Autodesk Fusion 360 part; units mm, degrees
sketch "Esquisse1" plane through (0, 0, 0) normal (0, 0, 1) x (1, 0, 0)
  line L0 (4.3054, 30) -> (67.3054, 30)
  line L1 (67.3054, 30) -> (67.3054, 12.25)
  line L2 (67.3054, 12.25) -> (4.3054, 12.25)
  line L3 (4.3054, 12.25) -> (4.3054, 30)
  dimension "d1" = 63
  dimension "d2" = 17.75
extrude "Extrusion1" add sketch "Esquisse1" along normal blind 1
sketch "Esquisse2" plane through (0, 0, 1) normal (0, 0, 1) x (-1, 0, 0)
  line L0 (-4.3054, -12.25) -> (-67.3054, -12.25)
  line L1 (-67.3054, -12.25) -> (-67.3054, -30)
  line L2 (-67.3054, -30) -> (-4.3054, -30)
  line L3 (-4.3054, -30) -> (-4.3054, -12.25)
  line L4 (-4.3054, -12.95) -> (-6.3054, -12.95)
  line L5 (-6.3054, -12.95) -> (-6.3054, -29.3)
  line L6 (-6.3054, -29.3) -> (-4.3054, -29.3)
  line L7 (-4.3054, -29.3) -> (-4.3054, -12.95)
  line L8 (-67.3054, -21.125) -> (-4.3054, -21.125) construction
  dimension "d5" = 16.35
  dimension "d8" = 2
extrude "Extrusion2" add sketch "Esquisse2" along normal blind 1 contours L3 L4 L5 L6 L7
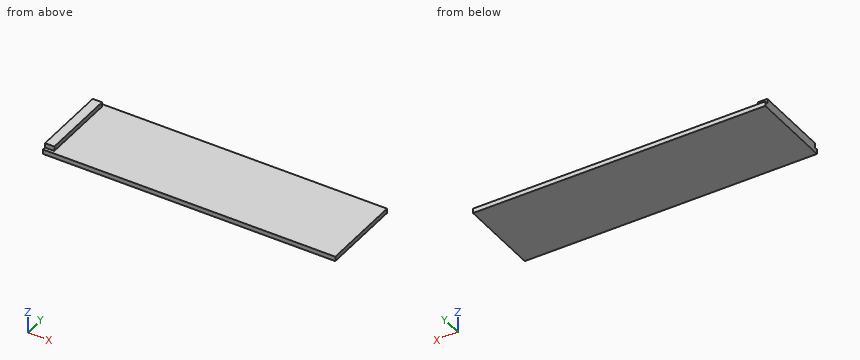
Geometry check sheet. Reference: the model listing, model coordinates, mm. Round coordinates to 2 decimals unless told otherwise and drop trailing zeros. Loops run counter-clockwise (first coordinate to the right, second up) from the corner with the lowest first, then second, coordinate; pieces in that order, holes last. Notation, with made-up numbers: (-14, 62.5) - (-6, 62.5) arc R32 ccw to (-6, 94.5) - close; hole circle Ø5 at (64, 36.25). An arc over 180 degrees is marked (long way). One line per question, with ' | ' between items. Start each with the question number.
1. Cross-section at C-C on x = 29. Record the cut outline in (y, z), then the cut area to 4 significant figures.
2. Depth check by flat-ended pin: pin 1 (0.8 mm diameter, centred on y = 20.5, z = 1.5, fed in from +X); pin 2 (9 mm diameter, centred on x = 44.5, y = 20, fed in from +Z); pin 3 (0.8 mm diameter, centred on x = 5.5, z = 1.5, fed in from +Y). Enter the tip coordinate at first touch or a pass-through.
3. Scan lines: line 1 (Z direction, x = 35, y = 27.75); line 2 (X direction, y = 15.25, z = 1.2). Record each from-to range of solid material in increasing order. Write a range as [from, to].
4. Cross-section at A-A on y = 13.5. Record the cut outline in (x, z).
5. Cross-section at B-B on z = 1.3. Record the cut outline in (x, y).
Taken from the geometry:
1) outline: (12.25, 0) - (30, 0) - (30, 1) - (12.25, 1) - close | area: 17.75 mm²
2) pin 1: x = 6.31 | pin 2: z = 1 | pin 3: y = 29.3
3) line 1: [0, 1] | line 2: [4.31, 6.31]
4) outline: (4.31, 0) - (67.31, 0) - (67.31, 1) - (6.31, 1) - (6.31, 2) - (4.31, 2) - close
5) outline: (4.31, 12.95) - (6.31, 12.95) - (6.31, 29.3) - (4.31, 29.3) - close
